Part model, mm, in its own coordinate system. Face numbers are marked on the shaded views. A direction names the side the tool comes from. Round coordinates to 2 decimals unless told otherwise and drop trailing zeros. Write each loop counter-clockwise with the first axis right and the second up, starting at its lowest first coordinate (ties: lowest second). Pieces come first, ordered by that corner, then holes. Notation, with made-up numbers: (-2.5, 2.25) -> (44.5, 2.25) arc R33 cw to (44.5, 33.25) -> close; hole circle Ø4 at (84.5, -38). An arc over 180 degrees is marked (long way). Return JSON: item names as keys, results as strings. Group by question number.
(1) Saw through at C-C (z = 2). List the corners of the cut face in (x, y).
(2) Drill centre lines: L1, parallel to Y at x = -7, z = 0; L2, parallel to Z at x = -8.3, y = 1; L3, parallel to X at y = 0.5, z = -5.75. Where is each one in solid material? Low to high. Write a range as from..to.
(3) Saw through at D-D (x = 8.5). List the corners of the cut face in (y, z), plus the area to 3 significant figures.
(4) Saw through at A-A (x = -8.3). List the corners of the cut face in (y, z), plus the area to 3 significant figures.
(5) Saw through at B-B (x = -5.5). List the corners of the cut face in (y, z), plus the area to 3 significant figures.
(6) Tool access for the marked faces 1, 2, 3 and 4: list every direction of +Z, -Z, +X, -X, +Y, -Y with a clear straight run to the whole face (end or side of a thin tool).
(7) Mould opens along Y. For the marked faces 5, 6 and 7 say: +Y half, -Y half, draft (parallel to the pull), parting line (faces both ways), or undercut.
(8) Drop flat-ended pins along their axis: pin 1 Ø2 at (y, z) = (-5, 2) entering from -X; pin 2 Ø0.9 at (x, y) = (-7.5, -10.5) entering from -Z; pin 3 Ø0.9 at (y, z) = (-11, -1.5) entering from +X. Give the stop position or say it passes through.
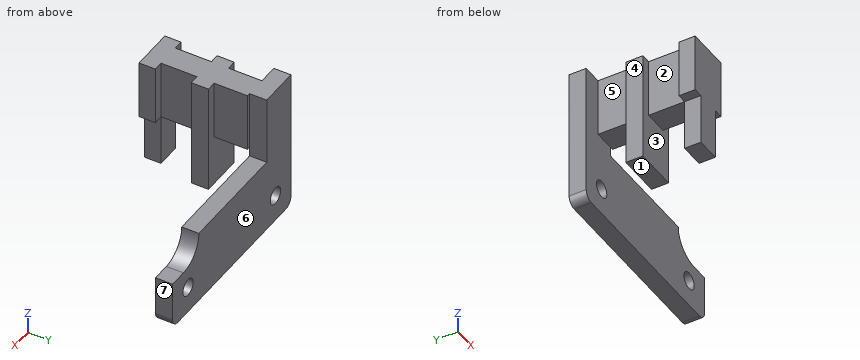
from build123d import *

# Parameters (mm, degrees)
SKETCH1_R           = 1
BOSS_EXTRUDE1_DEPTH = 2
BOSS_EXTRUDE2_START = 8
BOSS_EXTRUDE2_DEPTH = 6.9
SKETCH3_W           = 2.8
SKETCH3_H           = 1.9
SKETCH3_W_2         = 5
SKETCH3_H_2         = 2
BOSS_EXTRUDE3_DEPTH = 12.9


with BuildPart() as part:
    # Sketch1 → Boss-Extrude1 (new body)
    with BuildSketch(Plane(origin=(0, 0, 0), x_dir=(1, 0, 0), z_dir=(0, 1, 0))):
        with BuildLine():
            Line((11.7, 3), (11.7, 7.6))
            ThreePointArc((11.7, 7.6), (11.407106781, 8.307106781), (10.7, 8.6))
            Line((10.7, 8.6), (-10.3, 8.6))
            ThreePointArc((-10.3, 8.6), (-11.007106781, 8.307106781), (-11.3, 7.6))
            Line((-11.3, 7.6), (-11.3, -8))
            Line((-11.3, -8), (-6.6, -8))
            Line((-6.6, -8), (-6.6, 0))
            Line((-6.6, 0), (6.6, 0))
            ThreePointArc((6.6, 0), (7.478679656, 2.121320344), (9.6, 3))
            Line((9.6, 3), (11.7, 3))
        make_face()
        with Locations((8.7, 5.469565217)):
            Circle(SKETCH1_R, mode=Mode.SUBTRACT)
        with Locations((-8.3, 5.469565217)):
            Circle(SKETCH1_R, mode=Mode.SUBTRACT)
    extrude(amount=BOSS_EXTRUDE1_DEPTH)

    # Sketch2 → Boss-Extrude2 (add)
    with BuildSketch(Plane.XY.offset(BOSS_EXTRUDE2_START)):
        Polygon((-9, -10.1), (-9, 0), (-6.2, 0), (-6.2, -10.1), (-5.1, -10.1), (-5.1, -12), (-10.1, -12), (-10.1, -10.1), align=None)
    extrude(amount=-BOSS_EXTRUDE2_DEPTH)

    # Sketch3 → Boss-Extrude3 (add)
    with BuildSketch(Plane.XY.offset(8)):
        with Locations((-7.6, -11.05)):
            Rectangle(SKETCH3_W, SKETCH3_H)
        with Locations((-7.6, -4.9)):
            Rectangle(SKETCH3_W_2, SKETCH3_H_2)
    extrude(amount=-BOSS_EXTRUDE3_DEPTH)


solid = part.part
Computed values:
{
 "1": {"outline": "(-11.3, 0) -> (-9, 0) -> (-9, -3.9) -> (-10.1, -3.9) -> (-10.1, -5.9) -> (-9, -5.9) -> (-9, -10.1) -> (-10.1, -10.1) -> (-10.1, -12) -> (-5.1, -12) -> (-5.1, -10.1) -> (-6.2, -10.1) -> (-6.2, -5.9) -> (-5.1, -5.9) -> (-5.1, -3.9) -> (-6.2, -3.9) -> (-6.2, 0) -> (-6.6, 0) -> (-6.6, 2) -> (-11.3, 2) -> close"},
 "2": {"L1": "-12..-10.1, -5.9..-3.9, 0..2", "L2": "-8.6..-6.47, -4.47..8", "L3": "-11.3..-9.26, -7.34..7.74, 9.66..11.7"},
 "3": {"outline": "(0, -8.6) -> (2, -8.6) -> (2, -6.45) -> (0, -6.45) -> close; (0, -4.49) -> (2, -4.49) -> (2, -2.79) -> (0, -2.79) -> close", "area": "7.70 mm2"},
 "4": {"outline": "(-12, -4.9) -> (-10.1, -4.9) -> (-10.1, 1.1) -> (-5.9, 1.1) -> (-5.9, -4.9) -> (-3.9, -4.9) -> (-3.9, 1.1) -> (0, 1.1) -> (0, -4.47) -> (2, -4.47) -> (2, 8) -> (-12, 8) -> close; (0, -8.6) -> (2, -8.6) -> (2, -6.47) -> (0, -6.47) -> close", "area": "135 mm2"},
 "5": {"outline": "(-12, 1.1) -> (-10.1, 1.1) -> (-10.1, 8) -> (-12, 8) -> close; (-5.9, -4.9) -> (-3.9, -4.9) -> (-3.9, 8) -> (-5.9, 8) -> close; (0, -8.6) -> (2, -8.6) -> (2, 0) -> (0, 0) -> close", "area": "56.1 mm2"},
 "6": {"face 1": "-Z, +X, -X, -Y", "face 2": "+Z, -Z, -X", "face 3": "-Z", "face 4": "+Z, -Z, -X, -Y"},
 "7": {"face 5": "undercut", "face 6": "+Y half", "face 7": "draft"},
 "8": {"pin 1": "x = -10.1", "pin 2": "z = -4.9", "pin 3": "x = -6.2"}
}
